Read the model definition and answer for the solid it produces. Units are mm, in the model's axes. A direction names the side the tool comes from. Coordinates: 2 decimals unless noted, no trailing zeros. Loops run counter-clockwise (first coordinate to the right, second up) from the corner with the lowest first, then second, coordinate; pieces in that order, holes last. Notation, with made-up numbers: (-22.5, 84.25) - (25.5, 84.25) arc R26 ccw to (25.5, 117.25) - close; hole circle Ø1 at (46.25, -32). An arc over 180 degrees is marked (long way). Use one line per item in the form item = value. Start each with the question number.
1) The mould has two halves that part along X. Classify faces 1 (the face through (0, -7.23, 1)), 2 (the face through (-21, 0, -1)), 3 (the face through (0, 0, -1.5)), 4 (the face through (21, 0, -1)): released by +X, released by -X, zero draft, split by the parting line, or undercut.
2) A cutting plane is placed at A-A (z = 2.75). Give the vertices of the cut face in (x, y).
3) A cutting plane is placed at C-C (y = -3.5). Give the vertices of the cut face in (x, z).
4) Each of these flat-tipped pins is pushed along its axis until it touches: P1, Ø0.6, axis at x = -5, z = 4, coming from the +Y side; P2, Ø3, axis at y = -7, z = -9.5, coming from the +X side; P3, Ø1.5, axis at y = 5.5, z = -5.5, coming from the +X side. Where does it stop, or does it pass through?
5) Which of the six approach directions +Z, -Z, +X, -X, +Y, -Y give full straight-line access (tool end or side, diameter ignored) to faces 5 (the face through (0, -9.77, 1)), 6 (the face through (11, 0, -13)), 7 (the face through (0, 8, -3.5)), 8 (the face through (0, -10, -1)), 9 (the face through (6.35, -9, 1))?
6) A cutting plane is placed at B-B (x = -18.8). Give the vertices of the cut face in (y, z), and give its area (3 significant figures).
7) A cutting plane is placed at D-D (x = 11.25). Give the vertices of the cut face in (y, z).
8) Consider line 1 (Y direction, x = -18.8, z = -0.4); line 2 (X direction, y = -0.25, z = -10); line 3 (Y direction, x = -11.25, z = -13.05). Determine where each line is inside the solid, lowest interval first.
from build123d import *

# Parameters (mm, degrees)
CROQUIS1_W                   = 42
CROQUIS1_H                   = 20
CROQUIS1_R                   = 1.5
SALIENTE_EXTRUIR1_DEPTH      = 1.5
CROQUIS2_R                   = 8
SALIENTE_EXTRUIR2_DEPTH      = 12
CROQUIS3_R                   = 6.5
CORTAR_EXTRUIR1_DEPTH        = 0.5
CROQUIS5_W                   = 0.5
CROQUIS5_H                   = 0.5
SALIENTE_EXTRUIR3_DEPTH      = 8.5
SALIENTE_EXTRUIR3_DEPTH_BACK = 3
CROQUIS6_W                   = 12.7
CROQUIS6_H                   = 2.54
SALIENTE_EXTRUIR4_DEPTH      = 2
SALIENTE_EXTRUIR5_DEPTH      = 4
SALIENTE_EXTRUIR6_DEPTH      = 2


with BuildPart() as part:
    # Croquis1 → Saliente-Extruir1 (new body)
    with BuildSketch(Plane.XY):
        Rectangle(CROQUIS1_W, CROQUIS1_H)
        with Locations((-18.8, 7.8)):
            Circle(CROQUIS1_R, mode=Mode.SUBTRACT)
        with Locations((18.8, -7.8)):
            Circle(CROQUIS1_R, mode=Mode.SUBTRACT)
    extrude(amount=-SALIENTE_EXTRUIR1_DEPTH)

    # Croquis2 → Saliente-Extruir2 (add)
    with BuildSketch(Plane(origin=(0, 0, -1.5), x_dir=(-1, 0, 0), z_dir=(0, 0, -1))):
        with Locations((-11.25, 0)):
            Circle(CROQUIS2_R)
        with Locations((11.25, 0)):
            Circle(CROQUIS2_R)
    extrude(amount=SALIENTE_EXTRUIR2_DEPTH)

    # Croquis3 → Cortar-Extruir1 (cut)
    with BuildSketch(Plane(origin=(0, 0, -13.5), x_dir=(-1, 0, 0), z_dir=(0, 0, -1))):
        with Locations((-11.25, 0)):
            Circle(CROQUIS3_R)
        with Locations((11.25, 0)):
            Circle(CROQUIS3_R)
    extrude(amount=-CORTAR_EXTRUIR1_DEPTH, mode=Mode.SUBTRACT)

    # Croquis5 → Saliente-Extruir3 (add, two sides)
    with BuildSketch(Plane.XY) as saliente_extruir3_sk:
        with Locations((0, -8.5)):
            Rectangle(CROQUIS5_W, CROQUIS5_H)
        with Locations((-2.54, -8.5)):
            Rectangle(CROQUIS5_W, CROQUIS5_H)
        with Locations((-5.08, -8.5)):
            Rectangle(CROQUIS5_W, CROQUIS5_H)
        with Locations((2.54, -8.5)):
            Rectangle(CROQUIS5_W, CROQUIS5_H)
        with Locations((5.08, -8.5)):
            Rectangle(CROQUIS5_W, CROQUIS5_H)
    extrude(amount=SALIENTE_EXTRUIR3_DEPTH)
    extrude(saliente_extruir3_sk.sketch, amount=-SALIENTE_EXTRUIR3_DEPTH_BACK)

    # Croquis6 → Saliente-Extruir4 (add)
    with BuildSketch(Plane.XY):
        with Locations((0, -8.5)):
            Rectangle(CROQUIS6_W, CROQUIS6_H)
    extrude(amount=SALIENTE_EXTRUIR4_DEPTH)

    # Croquis7 → Saliente-Extruir5 (add)
    with BuildSketch(Plane(origin=(0, 0, -1.5), x_dir=(-1, 0, 0), z_dir=(0, 0, -1))):
        with BuildLine():
            Line((-2.5, -7), (0, -7))
            Line((0, -7), (2.5, -7))
            ThreePointArc((2.5, -7), (0, -4.5), (-2.5, -7))
        make_face()
    extrude(amount=SALIENTE_EXTRUIR5_DEPTH)

    # Croquis8 → Saliente-Extruir6 (add)
    with BuildSketch(Plane(origin=(0, 0, -1.5), x_dir=(-1, 0, 0), z_dir=(0, 0, -1))):
        with BuildLine():
            Line((-1.5, 9.5), (1.5, 9.5))
            ThreePointArc((1.5, 9.5), (2.5, 7.5), (1.5, 5.5))
            Line((1.5, 5.5), (-1.5, 5.5))
            ThreePointArc((-1.5, 5.5), (-2.5, 7.5), (-1.5, 9.5))
        make_face()
    extrude(amount=SALIENTE_EXTRUIR6_DEPTH)


solid = part.part
Found:
q1.face_1 = zero draft
q1.face_2 = released by -X
q1.face_3 = undercut
q1.face_4 = released by +X
q2.outline = (-5.33, -8.75) - (-4.83, -8.75) - (-4.83, -8.25) - (-5.33, -8.25) - close; (-2.79, -8.75) - (-2.29, -8.75) - (-2.29, -8.25) - (-2.79, -8.25) - close; (-0.25, -8.75) - (0.25, -8.75) - (0.25, -8.25) - (-0.25, -8.25) - close; (2.29, -8.75) - (2.79, -8.75) - (2.79, -8.25) - (2.29, -8.25) - close; (4.83, -8.75) - (5.33, -8.75) - (5.33, -8.25) - (4.83, -8.25) - close
q3.outline = (-21, -1.5) - (-18.44, -1.5) - (-18.44, -13.5) - (-16.73, -13.5) - (-16.73, -13) - (-5.77, -13) - (-5.77, -13.5) - (-4.06, -13.5) - (-4.06, -1.5) - (4.06, -1.5) - (4.06, -13.5) - (5.77, -13.5) - (5.77, -13) - (16.73, -13) - (16.73, -13.5) - (18.44, -13.5) - (18.44, -1.5) - (21, -1.5) - (21, 0) - (-21, 0) - close
q4.P1 = -8.25
q4.P2 = 17.06
q4.P3 = 17.69
q5.face_5 = +Z, +X, -X, -Y
q5.face_6 = -Z
q5.face_7 = -Z, +Y
q5.face_8 = +Z, -Z, +X, -X, -Y
q5.face_9 = +Z, +X, +Y, -Y
q6.outline = (-10, -1.5) - (-2.65, -1.5) - (-2.65, -13.5) - (2.65, -13.5) - (2.65, -1.5) - (6.3, -1.5) - (6.3, 0) - (-10, 0) - close; (9.3, -1.5) - (10, -1.5) - (10, 0) - (9.3, 0) - close
q6.area = 89.0 mm^2
q7.outline = (-10, -1.5) - (-8, -1.5) - (-8, -13.5) - (-6.5, -13.5) - (-6.5, -13) - (6.5, -13) - (6.5, -13.5) - (8, -13.5) - (8, -1.5) - (10, -1.5) - (10, 0) - (-10, 0) - close
q8.line_1 = -10 to 6.3, 9.3 to 10
q8.line_2 = -19.25 to -3.25, 3.25 to 19.25
q8.line_3 = -8 to -6.5, 6.5 to 8
